CAD build for the part. Positions are in the model's coordinates, mm. A direction names the side the tool comes from. Round coordinates to 2 decimals unless told otherwise and drop trailing zeros. Loops run counter-clockwise (first coordinate to the right, second up) from the corner with the lowest first, then second, coordinate; pieces in that order, holes last. Notation, with made-up numbers: M -26.5,-36.5 L -13.5,-36.5 A30 cw -13.5,-8.5 Z; hole C -34,13 d6. An arc over 180 degrees is marked long. Use a Markdown table: item, result. Add a question column.
(1) Flat gauge pins, fed straight in: P1, Ø9, axis at x = 0, y = 7, coming from the +Z side; P2, Ø6, axis at y = 8.5, z = 7, coming from the -X side; P3, Ø5, axis at x = 13, z = 11.5, coming from the +Y side; P4, Ø6, axis at x = 8.5, z = 5.5, coming from the +Y side. Where does each tip first touch, or does it go through?
(2) Wall check: L1, parallel to Y at x = 0, z = 7.5; L2, parallel to X at y = 7, z = 5.5; L3, parallel to Y at x = 8, z = 5.25. Give the ranges that are in metal, low to high.
(3) Band-saw the part on A-A, the plane y = 3. Write the cut outline in (x, z), and give its area (3 significant figures).
(4) Two-plate mould, pull along X, no slides. Class faces 4 (the face through (20, -1, 10)), 5 (the face through (-7, 4, 5)), 6 (the face through (-0.651, 11.957, 4.93)), 7 (the face through (0, 0, 12)): released by +X, released by -X, zero draft, split by the parting line, or undercut.
(5) Band-saw the part on D-D, the plane x = -13.5. Write the cut outline in (y, z), and give its area (3 significant figures).
(6) Band-saw the part on C-C, the plane x = 0. Write the cut outline in (y, z), and give its area (3 significant figures).
(7) Band-saw the part on B-B, the plane z = 7.75. Write the cut outline in (x, y).
(8) Which spindle directions (+Z, -Z, +X, -X, +Y, -Y) get a long thin tool onto all of the face, cutting with end or side? Do faces 1 (the face through (7, 3, 5)), 2 (the face through (0, 1, 0)), 3 (the face through (-3, 2, 10)). Say none if no direction does.
from build123d import *

# Parameters (mm, degrees)
F0_R     = 5
F1_DEPTH = 20
F2_R     = 2.75
F3_DEPTH = 2
F5_DEPTH = 10


with BuildPart() as f1:
    # F0 (on Top) → F1 (new body)
    with BuildSketch(Plane.XY):
        Polygon((-20, -2), (20, -2), (20, 0), (7, 0), (0, 0), (-7, 0), (-20, 0), align=None)
        with BuildLine():
            Line((0, 0), (7, 0))
            Line((7, 0), (7, 7))
            ThreePointArc((7, 7), (4.949747, 2.050253), (0, 0))
        make_face()
        with BuildLine():
            Line((-7, 7), (-7, 0))
            Line((-7, 0), (0, 0))
            ThreePointArc((0, 0), (-4.949747, 2.050253), (-7, 7))
        make_face()
        with BuildLine():
            ThreePointArc((-7, 7), (-4.949747, 2.050253), (0, 0))
            ThreePointArc((0, 0), (4.949747, 2.050253), (7, 7))
            ThreePointArc((7, 7), (0, 14), (-7, 7))
        make_face()
        with Locations((0, 7)):
            Circle(F0_R, mode=Mode.SUBTRACT)
    extrude(amount=F1_DEPTH)

    # F2 (on face) → F3 (cut, through all)
    with BuildSketch(Plane(origin=(0, 0, 0), x_dir=(-1, 0, 0), z_dir=(0, 1, 0))):
        with Locations((-13.5, 10)):
            Circle(F2_R)
        with Locations((13.5, 10)):
            Circle(F2_R)
    extrude(amount=-F3_DEPTH, mode=Mode.SUBTRACT)

    # F4 (on face) → F5 (cut)
    with BuildSketch(Plane.XY.offset(20)):
        with BuildLine():
            Line((-7, 7), (-7, 0))
            Line((-7, 0), (7, 0))
            Line((7, 0), (7, 7))
            ThreePointArc((7, 7), (4.949747, 11.949747), (0, 14))
            ThreePointArc((0, 14), (-4.949747, 11.949747), (-7, 7))
        make_face()
        with BuildLine():
            Line((-7, 14), (-7, 7))
            ThreePointArc((-7, 7), (-4.949747, 11.949747), (0, 14))
            Line((0, 14), (-7, 14))
        make_face()
        with BuildLine():
            ThreePointArc((0, 14), (4.949747, 11.949747), (7, 7))
            Line((7, 7), (7, 14))
            Line((7, 14), (0, 14))
        make_face()
    extrude(amount=-F5_DEPTH, mode=Mode.SUBTRACT)


solid = f1.part
Return value:
| question | item | result |
|---|---|---|
| 1 | P1 | through |
| 1 | P2 | x = -7 |
| 1 | P3 | y = 0 |
| 1 | P4 | y = 11.33 |
| 2 | L1 | -2 to 2, 12 to 14 |
| 2 | L2 | -7 to -5, 5 to 7 |
| 2 | L3 | -2 to 0 |
| 3 | outline | M -7,0 L -3,0 L -3,10 L -7,10 Z; M 3,0 L 7,0 L 7,10 L 3,10 Z |
| 3 | area | 80.0 mm^2 |
| 4 | face 4 | released by +X |
| 4 | face 5 | released by -X |
| 4 | face 6 | undercut |
| 4 | face 7 | zero draft |
| 5 | outline | M -2,0 L 0,0 L 0,7.25 L -2,7.25 Z; M -2,12.75 L 0,12.75 L 0,20 L -2,20 Z |
| 5 | area | 29.0 mm^2 |
| 6 | outline | M -2,0 L 2,0 L 2,10 L 0,10 L 0,20 L -2,20 Z; M 12,0 L 14,0 L 14,10 L 12,10 Z |
| 6 | area | 80.0 mm^2 |
| 7 | outline | M -20,-2 L -15.08,-2 L -15.08,0 L -20,0 Z; M -11.92,-2 L 11.92,-2 L 11.92,0 L 7,0 L 7,7 A7 ccw -7,7 L -7,0 L -11.92,0 Z; M 15.08,-2 L 20,-2 L 20,0 L 15.08,0 Z; hole C 0,7 d10 |
| 8 | face 1 | +Z, -Z, +X, +Y |
| 8 | face 2 | -Z, +X, -X, +Y, -Y |
| 8 | face 3 | +Z, +X, -X, +Y |
